Answer from the drawing. Dimensions are ordinates in mm from the lowest x, y and z of the part. A direction names the side the tool comes from. Give positions to 0.01 mm unless a question says otherwise; leave off trailing zeros. Loops run counter-clockwise (first coordinate to the right, second up) from the corner with the lowest first, then second, coordinate; pieces in that order, holes last. Notation, with made-up numbers: M 8,40 L 63,40 A23 ccw 63,67 Z; hole C 30.5,-28 d5. An arc over 180 degrees is marked long. Return JSON: item names as keys, results as strings. Group by question number.
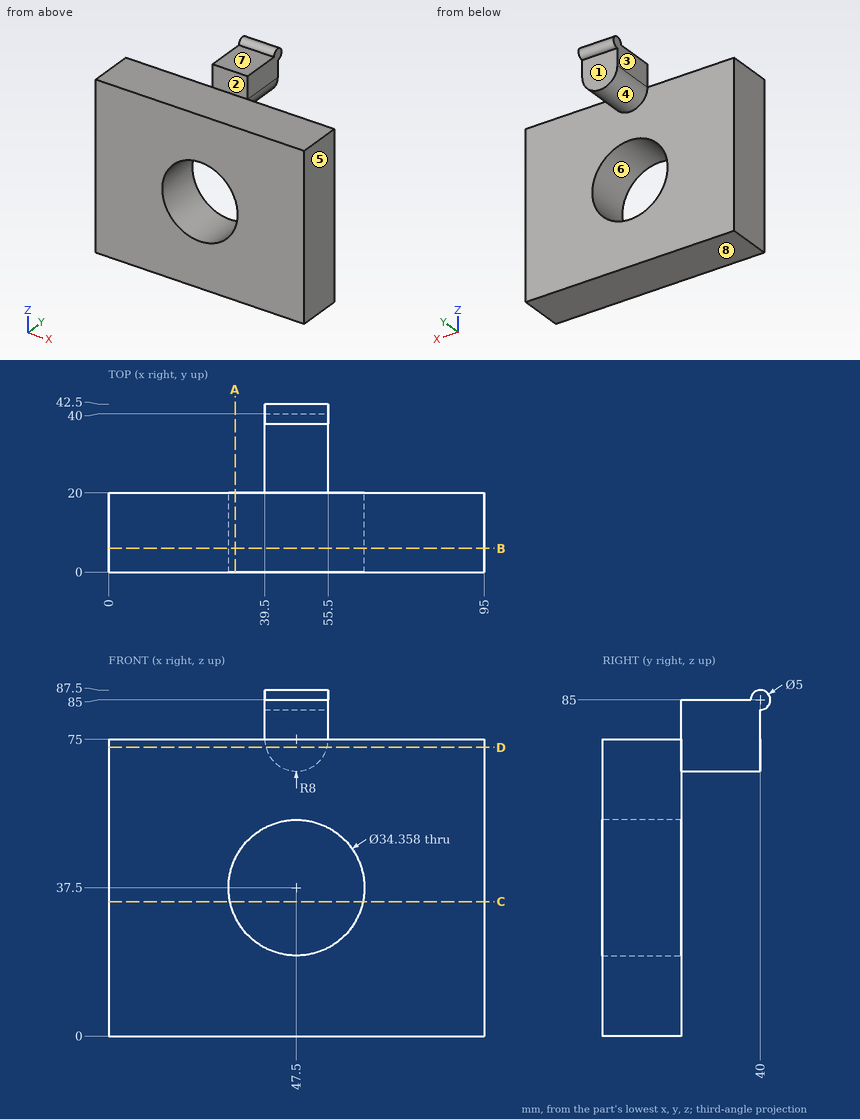
1. For the marked faces 1, 2, 3, 4 and 5, determine the directions among +Z, -Z, +X, -X, +Y, -Y from which every point of the face is accessible in a straight line to the end or side of a thin tool.
2. The mould has two halves that part along Z. Classify the marked faces 6, 7 and 8: +Z half, -Z half, draft (parallel to the pull), parting line (faces both ways), or undercut.
3. Find section A-A (x = 32). Write down the section's boundary in (y, z), and give its area (3 significant figures).
4. Find section D-D (z = 73). Write down the section's boundary in (x, y), and give its area (3 significant figures).
5. Find section C-C (z = 34). Write down the section's boundary in (x, y).
6. Straight lines are drawn through the part: line 1 along Z through (x, y) = (47, 6); line 2 along X through (y, z) = (9, 37); line 3 along Y through (x, z) = (73, 20.5). For each, find the intervals that lie inside material, in ascending order.
7. Find section B-B (y = 6). Write down the section's boundary in (x, z).
8. Flat-ended cylindrical pins translate along their axes: P1, Ø4, axis at x = 76, y = 17.5, coming from the +Z side; P2, Ø8, axis at x = 49, z = 73.5, coming from the +Y side; P3, Ø14, axis at y = 28, z = 79.5, coming from the -X side; P4, Ø6, axis at y = 36.5, z = 62.5, coming from the -X side. Find the tip coordinate at first contact, or state that the pin passes through.
Result:
{
 "1": {"face 1": "-Z, +X, -X, +Y", "face 2": "+Z, +X, -X, -Y", "face 3": "+Z, -Z, -X, +Y, -Y", "face 4": "-Z, +Y", "face 5": "+Z, -Z, +X, +Y, -Y"},
 "2": {"face 6": "undercut", "face 7": "+Z half", "face 8": "-Z half"},
 "3": {"outline": "M 0,0 L 20,0 L 20,30.09 L 0,30.09 Z; M 0,44.91 L 20,44.91 L 20,75 L 0,75 Z", "area": "1,200 mm2"},
 "4": {"outline": "M 0,0 L 95,0 L 95,20 L 55.25,20 L 55.25,40 L 39.75,40 L 39.75,20 L 0,20 Z", "area": "2,210 mm2"},
 "5": {"outline": "M 0,0 L 30.68,0 L 30.68,20 L 0,20 Z; M 64.32,0 L 95,0 L 95,20 L 64.32,20 Z"},
 "6": {"line 1": "z = 0 to 20.33, 54.67 to 75", "line 2": "x = 0 to 30.33, 64.67 to 95", "line 3": "y = 0 to 20"},
 "7": {"outline": "M 0,0 L 95,0 L 95,75 L 0,75 Z; hole C 47.5,37.5 d34.36"},
 "8": {"P1": "stops at z = 75", "P2": "stops at y = 40", "P3": "stops at x = 39.5", "P4": "passes through"}
}
